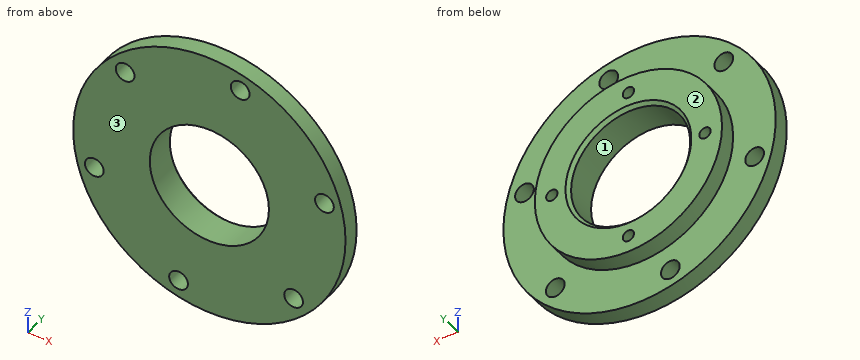
Autodesk Inventor part; units mm, degrees
ref_plane "YZ Plane" through (0, 0, 0) normal (1, 0, 0) x (0, 1, 0)
ref_plane "XZ Plane" through (0, 0, 0) normal (0, 1, 0) x (-1, 0, 0)
ref_plane "XY Plane" through (0, 0, 0) normal (0, 0, 1) x (1, 0, 0)
sketch "Эскиз1" plane through (0, 0, 0) normal (0, 0, 1) x (1, 0, 0)
  line L0 (0, 0) -> (0, -30.9602)
  line L1 (35, 0) -> (35, -20)
  line L2 (35, -20) -> (80, -20)
  line L3 (80, -20) -> (80, -10)
  line L4 (80, -10) -> (55, -10)
  line L5 (55, -10) -> (55, 0)
  line L6 (55, 0) -> (35, 0)
  dimension "d0" = 70
  dimension "d1" = 110
  dimension "diam_out_plate" = 160
  dimension "d3" = 20
  dimension "d4" = 10
revolve "Вращение1" add sketch "Эскиз1" angle 360 about axis through (0, 0, 0) along (0, -1, 0)
sketch "Эскиз2" plane through (0, 0, 0) normal (0, 1, 0) x (1, 0, 0)
  circle A0 centre (0, 0) radius 35
  circle A1 centre (0, 0) radius 55
  point P0 (0, 45)
  dimension "d6" = 45
hole "Отверстие1" at (0, 0, -45) direction (0, -1, 0) diameter 6.647 depth 18 tip angle 118
pattern_circular "Круговой массив1" count 4 over 360 about axis through (0, -10, 0) along (0, -1, 0) of "Отверстие1"
sketch "Эскиз3" plane through (0, -10, 0) normal (0, 1, 0) x (1, 0, 0)
  circle A0 centre (0, 0) radius 55
  circle A1 centre (0, 0) radius 80
  circle A2 centre (0, 0) radius 80
  line L0 (0, 80) -> (0, 0)
  line L1 (0, 0) -> (49.4975, 49.4975) construction
  dimension "d17" = 70
  dimension "d18" = 45
hole "Отверстие2" at (49.4975, -10, -49.4975) direction (0, -1, 0) diameter 11 end through all
pattern_circular "Круговой массив2" count 6 over 360 about axis through (0, -10, 0) along (0, -1, 0) of "Отверстие2"
chamfer "Фаска2" distance 2 angle 45 1 edges at (-35, 0, 0)
properties part number "плашка"
Verification items for the finished model (mm, model axes). Face numbers are marked on the shaded views. Coordinates: 2 decimals unless noted, no trailing zeros. Write each loop counter-clockwise with the first axis right and the second up, starting at its lowest first coordinate (ties: lowest second). Pieces come first, ordered by that corner, then holes. Notation, with made-up numbers: M 34.25,58 L 91.25,58 A32 ccw 91.25,97 Z; hole C -19,62.5 d9. An arc over 180 degrees is marked long. Use a Markdown table: item, result.
Q1. Sectioned sample at C-C, the plane x = 39. Record the boundary of the cut face in (y, z), plus the area to 3 significant figures.
Reply:
| item | result |
|---|---|
| outline | M -20,-69.85 L -10,-69.85 L -10,-38.78 L 0,-38.78 L 0,38.78 L -10,38.78 L -10,69.85 L -20,69.85 Z |
| area | 2,170 mm² |
Q2. Sectioned sample at A-A, the plane y = -6.75. Record the boundary of the cut face in (x, z).
Reply:
| item | result |
|---|---|
| outline | C 0,0 d110; hole C -45,0 d6.65; hole C 0,0 d70; hole C 0,-45 d6.65; hole C 0,45 d6.65; hole C 45,0 d6.65 |
Q3. Thickness scan on line 1 (X direction, y = -12, z = -45); line 2 (Z direction, x = 47, y = -16.25); line 3 (Y direction, x = -21.5, z = -60.5). Record the ranges inside material, lowest first.
Reply:
| item | result |
|---|---|
| line 1 | x = -66.14 to -3.32, 3.32 to 46.33, 52.66 to 66.14 |
| line 2 | z = -64.74 to -54.4, -44.6 to -2.65, 2.65 to 64.74 |
| line 3 | y = -20 to -10 |
Q4. Go/stop test with flat-tipped pins: P1, Ø5, axis at y = -12, z = 56, coming from the -X side; P2, Ø17.5, axis at x = 67.61, z = 18.12, coming from the +Y side; P3, Ø12, axis at y = -7.5, z = -48.5, coming from the -X side. Record where each tip stops, or that it passes through.
Reply:
| item | result |
|---|---|
| P1 | stops at x = -59.48 |
| P2 | stops at y = -10 |
| P3 | stops at x = -67.43 |
Q5. Sectioned sample at D-D, the plane z = -57.5. Record the boundary of the cut face in (x, y).
Reply:
| item | result |
|---|---|
| outline | M -55.62,-20 L 55.62,-20 L 55.62,-10 L -55.62,-10 Z |
Q6. Sectioned sample at B-B, the plane x = 18.5. Count the separate pieces of the cut face and the enclosed holes in it, plus the area to 3 significant figures.
Reply:
| item | result |
|---|---|
| separate pieces | 3 |
| enclosed holes | 0 |
| area | 1,290 mm² |
Q7. Draft check along Y on the marked faces 1, 2 and 3. Enter one of: +Y half, -Y half, draft (parallel to the pull), parting line (faces both ways), or undercut.
Reply:
| item | result |
|---|---|
| face 1 | draft |
| face 2 | +Y half |
| face 3 | -Y half |
